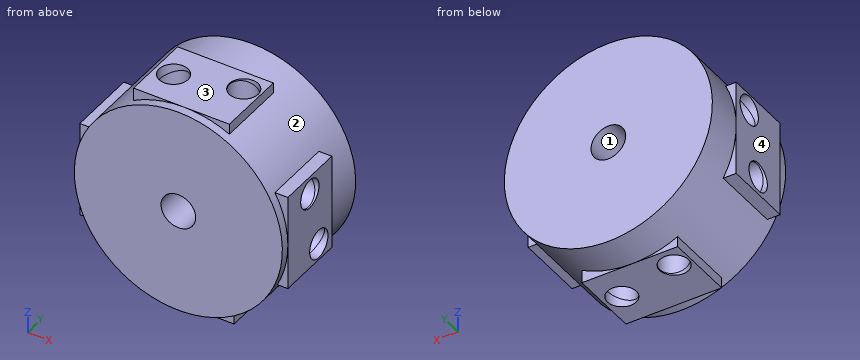
from build123d import *

# Parameters (mm, degrees)
ESQUISSE1_R                  = 18
ESQUISSE1_R_2                = 3
BOSS_EXTRU_1_DEPTH           = 20
BOSS_EXTRU_2_REACH           = 46.944
BOSS_EXTRU_2_END_RADIUS      = 18
ESQUISSE2_W                  = 16.575364331
ESQUISSE2_H                  = 12
ESQUISSE2_R                  = 2.5
ESQUISSE3_R                  = 2.5
ENL_V_MAT_EXTRU_1_DEPTH      = 8
R_P_TITION_CIRCULAIRE1_COUNT = 4


with BuildPart() as part:
    # Esquisse1 → Boss.-Extru.1 (new body)
    with BuildSketch(Plane(origin=(0, 0, 0), x_dir=(1, 0, 0), z_dir=(0, 1, 0))):
        with Locations(Location((0, 0, 0), (0, 0, 270))):
            Circle(ESQUISSE1_R)
        with Locations(Location((0, 0, 0), (0, 0, 270))):
            Circle(ESQUISSE1_R_2, mode=Mode.SUBTRACT)
    extrude(amount=BOSS_EXTRU_1_DEPTH)

    # Boss.-Extru.2: up to this cylinder (the profile starts outside it)
    boss_extru_2_end = Plane(origin=(0, 7.199085, 0), z_dir=(0, -1, 0)) * Cylinder(BOSS_EXTRU_2_END_RADIUS, 130.888, mode=Mode.PRIVATE)
    # Esquisse2 → Boss.-Extru.2 (add, up to the surface)
    with BuildSketch(Plane.ZY.offset(18), mode=Mode.PRIVATE) as boss_extru_2_sk1:
        with Locations((-0.409721573, 7.5)):
            Rectangle(ESQUISSE2_W, ESQUISSE2_H)
        with Locations((-5.58835764, 7.5)):
            Circle(ESQUISSE2_R, mode=Mode.SUBTRACT)
        with Locations((5.008479737, 9.946472677)):
            Circle(ESQUISSE2_R, mode=Mode.SUBTRACT)
    boss_extru_2_tool1 = extrude(boss_extru_2_sk1.sketch, amount=-BOSS_EXTRU_2_REACH, mode=Mode.PRIVATE) - boss_extru_2_end
    boss_extru_2 = boss_extru_2_tool1.solids().sort_by_distance((-18, 7.199085, -0.439188))[0] + boss_extru_2_tool1.solids().sort_by_distance((-18, 7.199085, -0.439188))[1]
    add(boss_extru_2)

    # Esquisse3 → Enlèv. mat.-Extru.1 (cut)
    with BuildSketch(Plane.ZY.offset(18)):
        with Locations((5.008479737, 9.946472677)):
            Circle(ESQUISSE3_R)
        with Locations((-5.58835764, 7.5)):
            Circle(ESQUISSE3_R)
    enl_v_mat_extru_1 = extrude(amount=-ENL_V_MAT_EXTRU_1_DEPTH, mode=Mode.SUBTRACT)

    # Répétition circulaire1: Boss.-Extru.2, Enlèv. mat.-Extru.1 ×4 about axis
    r_p_tition_circulaire1_axis = Axis((0, 0, 0), (0, 1, 0))
    add([boss_extru_2.rotate(r_p_tition_circulaire1_axis, i * 360 / R_P_TITION_CIRCULAIRE1_COUNT) for i in range(1, R_P_TITION_CIRCULAIRE1_COUNT)])
    add([enl_v_mat_extru_1.rotate(r_p_tition_circulaire1_axis, i * 360 / R_P_TITION_CIRCULAIRE1_COUNT) for i in range(1, R_P_TITION_CIRCULAIRE1_COUNT)], mode=Mode.SUBTRACT)


solid = part.part
Can you work these out from the model? Positions are in its coordinate system, mm. Face numbers are marked on the shaded views. Coordinates: 2 decimals unless noted, no trailing zeros. Write each loop counter-clockwise with the first axis right and the second up, starting at its lowest first coordinate (ties: lowest second). Pieces come first, ordered by that corner, then holes. Notation, with made-up numbers: (87, -25.75) - (101, -25.75) arc R31 cw to (101, -0.75) - close; hole circle Ø6 at (-14.5, 85). An arc over 180 degrees is marked (long way). Return JSON: item names as keys, results as strings. Group by question number.
Item 1: If we section it at B-B (z = 1.5): Write out the boundary of the cut face in (x, y).
Item 2: We'd pull the mould along X, two halves only. Please class the marked faces 1, 2, 3 and 4: pulls with the +X half, pulls with the -X half, needs draft (parallel to the pull), parting line crosses it, or undercut.
Item 3: I'm going to push flat-ended pins straight in: pin 1 Ø3 at (y, z) = (7.5, -5.59) entering from -X; pin 2 Ø0.9 at (x, y) = (-16.5, 9.5) entering from +Z; pin 3 Ø1 at (x, y) = (6.5, 9) entering from +Z. Where does each tip first touch, or does it pass through?
Item 4: If we section it at D-D (z = 7): Write out the boundary of the cut face in (x, y).
Item 5: Please list where these lines run through material, in increasing order: probe 1 along X at (y, z) = (9.5, 16); probe 2 along X at (y, z) = (12.75, 0); probe 3 along X at (y, z) = (8.25, 16).
Return value:
{
 "1": {"outline": "(-18, 1.5) - (-17.94, 1.5) - (-17.94, 0) - (-2.6, 0) - (-2.6, 20) - (-17.94, 20) - (-17.94, 13.5) - (-18, 13.5) - close; (2.6, 0) - (17.94, 0) - (17.94, 1.5) - (18, 1.5) - (18, 13.5) - (17.94, 13.5) - (17.94, 20) - (2.6, 20) - close"},
 "2": {"face 1": "undercut", "face 2": "parting line crosses it", "face 3": "needs draft", "face 4": "pulls with the -X half"},
 "3": {"pin 1": "stops at x = -10", "pin 2": "stops at z = 8.15", "pin 3": "stops at z = 10"},
 "4": {"outline": "(-18, 1.5) - (-16.58, 1.5) - (-16.58, 0) - (16.58, 0) - (16.58, 1.5) - (18, 1.5) - (18, 5.44) - (10, 5.44) - (10, 9.56) - (18, 9.56) - (18, 13.5) - (16.58, 13.5) - (16.58, 20) - (-16.58, 20) - (-16.58, 13.5) - (-18, 13.5) - (-18, 11.46) - (-10, 11.46) - (-10, 8.44) - (-18, 8.44) - close"},
 "5": {"probe 1": "x = -8.7 to -7.09, -4.09 to 2.55, 7.47 to 8.25", "probe 2": "x = -18 to -3, 3 to 18", "probe 3": "x = -8.7 to -7.97, -3.2 to 3.17, 6.84 to 8.25"}
}
